```python
from build123d import *

# Parameters (mm, degrees)
BOX_W          = 1
BOX_H          = 10
BOX_DEPTH      = 1
CYLINDER_R     = 2
CYLINDER_DEPTH = 10


with BuildPart() as cube:
    # Box → Box (new body)
    with BuildSketch(Plane(origin=(-0.5, -5, 0), x_dir=(1, 0, 0), z_dir=(0, 0, 1))):
        with Locations((0.5, 5)):
            Rectangle(BOX_W, BOX_H)
    extrude(amount=BOX_DEPTH)


with BuildPart() as cut:
    # Cone → Cone (revolve)
    with BuildSketch(Plane.XZ):
        Polygon((0, 0), (2.8, 0), (2, 2.2), (0, 2.2), align=None)
    revolve(axis=Axis((0, 0, 0), (0, 0, 1)))

    # Cut: cut Cube
    add(cube.part, mode=Mode.SUBTRACT)


with BuildPart() as fusion:
    # Cylinder → Cylinder (new body)
    with BuildSketch(Plane.XY.offset(2)):
        Circle(CYLINDER_R)
    extrude(amount=CYLINDER_DEPTH)

    # Fusion: union Cut
    add(cut.part)


solid = fusion.part
```
Input: part model. Units: mm. Frame: model coordinates. A direction names the side the tool comes from. Give positions to 0.01 mm unless a question says otherwise; leave off trailing zeros. Write each loop counter-clockwise with the first axis right and the second up, starting at its lowest first coordinate (ties: lowest second). Pieces come first, ordered by that corner, then holes. Notation, with made-up numbers: (33.5, -11) - (62.5, -11) arc R21 ccw to (62.5, 26) - close; hole circle Ø8 at (57.5, 31). An arc over 180 degrees is marked (long way). Write item = value, one per line. Start each with the question number.
1. Section query A-A, the plane y = 0. Output: boundary loops of the cut face in (x, z), then the cut area to 3 significant figures.
2. First-contact query: pin 1 Ø1 at (y, z) = (-1, 9.5) entering from -X; pin 2 Ø1.5 at (x, y) = (-0.5, 0) entering from -Z; pin 3 Ø2 at (y, z) = (1.5, 1.5) entering from +X; pin 4 Ø1.5 at (x, z) = (-1.5, 9.5) entering from -Y. Flat tips, straight axial feed; report the tip coordinate or a pass-through.
3. Mould query, pull axis X, two halves, no side actions, for faces 1 (the flat face through (0, 0, 1)), 2 (the cylindrical face through (0, -2, 7)), 3 (the flat face through (0, 0, 12)). Classes: released by +X, released by -X, zero draft, split by the parting line, or undercut.
4. Ray query, L1, parallel to Y at x = 0, z = 5.5; L2, parallel to Z at x = 1.65, y = -1.75. Return the intervals inside material, ascending.
5. Section query B-B, the plane x = 0. Output: boundary loops of the cut face in (y, z).
6. Section query C-C, the plane z = 2.5. Output: boundary loops of the cut face in (x, y), then the cut area to 3 significant figures.
7. Access query for faces 4 (the flat face through (-0.5, 0, 0.5)), 5 (the conical face through (-0.461, -2.077, 1.849)). Directions: +Z, -Z, +X, -X, +Y, -Y. A direction counts if a zero-diameter tool reaches every point of the face in a straight line with its end or side. Return the directions, or none.
Check sheet entries:
q1.outline = (-2.8, 0) - (-0.5, 0) - (-0.5, 1) - (0.5, 1) - (0.5, 0) - (2.8, 0) - (2, 2.2) - (2, 12) - (-2, 12) - (-2, 2.2) - close
q1.area = 48.8 mm2
q2.pin_1 = -1.94
q2.pin_2 = 0
q2.pin_3 = 2.38
q2.pin_4 = -1.85
q3.face_1 = undercut
q3.face_2 = split by the parting line
q3.face_3 = zero draft
q4.L1 = -2 to 2
q4.L2 = 0 to 1.09
q5.outline = (-2.44, 1) - (2.44, 1) - (2, 2.2) - (2, 12) - (-2, 12) - (-2, 2.2) - close
q6.outline = circle Ø4 at (0, 0)
q6.area = 12.6 mm2
q7.face_4 = -Z, +Y, -Y
q7.face_5 = +Z
